from build123d import *

# Parameters (mm, degrees)
SKETCH3_RX          = 5.624926532
SKETCH3_RY          = 3.004692616
SKETCH3_RX_2        = 9.556829234
SKETCH3_RY_2        = 4.328681477
SKETCH3_RX_3        = 8.492460802
SKETCH3_RY_3        = 4.684720213
SKETCH3_RX_4        = 5.848490675
SKETCH3_RY_4        = 3.57108896
SKETCH3_RX_5        = 14.471517628
SKETCH3_RY_5        = 10.662983723
BOSS_EXTRUDE2_DEPTH = 2.5


with BuildPart() as part:
    # Sketch3 → Boss-Extrude2 (new body)
    with BuildSketch(Plane(origin=(0, 0, 0), x_dir=(1, 0, 0), z_dir=(0, 1, 0))):
        Polygon((10.338651831, 158.825979178), (13.264554689, 163.800014037), (45.578225854, 148.199099997), (73.311205528, 123.503793754), (73.311205528, 113.306124028), (70.253487054, 110.248405554), (70.253487054, 91.907219464), (73.927331416, 81.033815485), (86.933442966, 42.539886198), (86.933442966, 30.301657501), (81.461542635, 24.829757171), (81.461542635, -24.829757171), (86.933442966, -30.301657501), (86.933442966, -42.539886198), (73.927331416, -81.033815485), (70.253487054, -91.907219464), (70.253487054, -110.248405554), (73.311205528, -113.306124028), (73.311205528, -123.503793754), (45.578225854, -148.199099997), (13.264554689, -163.800014037), (10.338651831, -158.825979178), (-10.338651831, -158.825979178), (-13.264554689, -163.800014037), (-45.578225854, -148.199099997), (-73.311205528, -123.503793754), (-73.311205528, -113.306124028), (-70.253487054, -110.248405554), (-70.253487054, -91.907219464), (-73.927331416, -81.033815485), (-86.933442966, -42.539886198), (-86.933442966, -30.301657501), (-81.461542635, -24.829757171), (-81.461542635, 24.829757171), (-86.933442966, 30.301657501), (-86.933442966, 42.539886198), (-73.927331416, 81.033815485), (-70.253487054, 91.907219464), (-70.253487054, 110.248405554), (-73.311205528, 113.306124028), (-73.311205528, 123.503793754), (-45.578225854, 148.199099997), (-13.264554689, 163.800014037), (-10.338651831, 158.825979178), align=None)
        with Locations(Location((11.385123615, 149.68538673), (0, 0, 83.157226587))):
            Ellipse(SKETCH3_RX, SKETCH3_RY, mode=Mode.SUBTRACT)
        with Locations(Location((33.692455497, 82.363006755), (0, 0, 39.093858886))):
            Ellipse(SKETCH3_RX_2, SKETCH3_RY_2, mode=Mode.SUBTRACT)
        with Locations(Location((44.895501329, 74.018669169), (0, 0, 39.093858886))):
            Ellipse(SKETCH3_RX_3, SKETCH3_RY_3, mode=Mode.SUBTRACT)
        with Locations(Location((66.355525512, 66.446955434), (0, 0, 82.221640152))):
            Ellipse(SKETCH3_RX_4, SKETCH3_RY_4, mode=Mode.SUBTRACT)
        with Locations(Location((-66.355525512, 66.446955434), (0, 0, 97.778359848))):
            Ellipse(SKETCH3_RX_4, SKETCH3_RY_4, mode=Mode.SUBTRACT)
        with Locations(Location((-44.895501329, 74.018669169), (0, 0, 140.906141114))):
            Ellipse(SKETCH3_RX_3, SKETCH3_RY_3, mode=Mode.SUBTRACT)
        with Locations(Location((-33.692455497, 82.363006755), (0, 0, 140.906141114))):
            Ellipse(SKETCH3_RX_2, SKETCH3_RY_2, mode=Mode.SUBTRACT)
        with Locations(Location((-11.385123615, 149.68538673), (0, 0, 96.842773413))):
            Ellipse(SKETCH3_RX, SKETCH3_RY, mode=Mode.SUBTRACT)
        with Locations(Location((-11.385123615, -149.68538673), (0, 0, -96.842773413))):
            Ellipse(SKETCH3_RX, SKETCH3_RY, mode=Mode.SUBTRACT)
        with Locations(Location((-33.692455497, -82.363006755), (0, 0, -140.906141114))):
            Ellipse(SKETCH3_RX_2, SKETCH3_RY_2, mode=Mode.SUBTRACT)
        with Locations(Location((-44.895501329, -74.018669169), (0, 0, -140.906141114))):
            Ellipse(SKETCH3_RX_3, SKETCH3_RY_3, mode=Mode.SUBTRACT)
        with Locations(Location((-66.355525512, -66.446955434), (0, 0, -97.778359848))):
            Ellipse(SKETCH3_RX_4, SKETCH3_RY_4, mode=Mode.SUBTRACT)
        with Locations(Location((66.355525512, -66.446955434), (0, 0, -82.221640152))):
            Ellipse(SKETCH3_RX_4, SKETCH3_RY_4, mode=Mode.SUBTRACT)
        with Locations(Location((44.895501329, -74.018669169), (0, 0, -39.093858886))):
            Ellipse(SKETCH3_RX_3, SKETCH3_RY_3, mode=Mode.SUBTRACT)
        with Locations(Location((33.692455497, -82.363006755), (0, 0, -39.093858886))):
            Ellipse(SKETCH3_RX_2, SKETCH3_RY_2, mode=Mode.SUBTRACT)
        with Locations(Location((11.385123615, -149.68538673), (0, 0, -83.157226587))):
            Ellipse(SKETCH3_RX, SKETCH3_RY, mode=Mode.SUBTRACT)
        with Locations(Location((0, 0), (0, 0, 90))):
            Ellipse(SKETCH3_RX_5, SKETCH3_RY_5, mode=Mode.SUBTRACT)
        Polygon((5.834875923, 128.014628126), (5.834875923, 107.44522339), (9.270194242, 107.44522339), (10.662983723, 103.716266976), (20.757785776, 101.069910811), (32.198995676, 111.76010755), (32.198995676, 123.503793754), (24.907753398, 123.503793754), (13.841173073, 132.585606956), (9.270194242, 132.585606956), align=None, mode=Mode.SUBTRACT)
        Polygon((41.941351313, 39.789061162), (51.486619053, 54.160218526), (55.402714886, 54.160218526), (58.163676153, 51.399257259), (58.163676153, 43.187167337), (66.355525512, 28.46204058), (66.355525512, 24.072820104), (62.259600832, 17.90608076), (47.849651346, 18.166894335), (41.941351313, 27.187750764), align=None, mode=Mode.SUBTRACT)
        Polygon((-41.941351313, 27.187750764), (-41.941351313, 39.789061162), (-51.486619053, 54.160218526), (-55.402714886, 54.160218526), (-58.163676153, 51.399257259), (-58.163676153, 43.187167337), (-66.355525512, 28.46204058), (-66.355525512, 24.072820104), (-62.259600832, 17.90608076), (-47.849651346, 18.166894335), align=None, mode=Mode.SUBTRACT)
        Polygon((-9.270194242, 132.585606956), (-5.834875923, 128.014628126), (-5.834875923, 107.44522339), (-9.270194242, 107.44522339), (-10.662983723, 103.716266976), (-20.757785776, 101.069910811), (-32.198995676, 111.76010755), (-32.198995676, 123.503793754), (-24.907753398, 123.503793754), (-13.841173073, 132.585606956), align=None, mode=Mode.SUBTRACT)
        Polygon((-5.834875923, -128.014628126), (-5.834875923, -107.44522339), (-9.270194242, -107.44522339), (-10.662983723, -103.716266976), (-20.757785776, -101.069910811), (-32.198995676, -111.76010755), (-32.198995676, -123.503793754), (-24.907753398, -123.503793754), (-13.841173073, -132.585606956), (-9.270194242, -132.585606956), align=None, mode=Mode.SUBTRACT)
        Polygon((-41.941351313, -39.789061162), (-51.486619053, -54.160218526), (-55.402714886, -54.160218526), (-58.163676153, -51.399257259), (-58.163676153, -43.187167337), (-66.355525512, -28.46204058), (-66.355525512, -24.072820104), (-62.259600832, -17.90608076), (-47.849651346, -18.166894335), (-41.941351313, -27.187750764), align=None, mode=Mode.SUBTRACT)
        Polygon((41.941351313, -27.187750764), (41.941351313, -39.789061162), (51.486619053, -54.160218526), (55.402714886, -54.160218526), (58.163676153, -51.399257259), (58.163676153, -43.187167337), (66.355525512, -28.46204058), (66.355525512, -24.072820104), (62.259600832, -17.90608076), (47.849651346, -18.166894335), align=None, mode=Mode.SUBTRACT)
        Polygon((9.270194242, -132.585606956), (5.834875923, -128.014628126), (5.834875923, -107.44522339), (9.270194242, -107.44522339), (10.662983723, -103.716266976), (20.757785776, -101.069910811), (32.198995676, -111.76010755), (32.198995676, -123.503793754), (24.907753398, -123.503793754), (13.841173073, -132.585606956), align=None, mode=Mode.SUBTRACT)
    extrude(amount=BOSS_EXTRUDE2_DEPTH)


solid = part.part
Geometry check sheet. Reference: the model listing, model coordinates, mm. A direction names the side the tool comes from. Give positions to 0.01 mm unless a question says otherwise; leave off trailing zeros.
(1) Release check for a two-part mould opening along Z. For faces 3 (the flat face through (-29.65, 1.23, -155.89)), 4 (the flat face through (-18, 2.5, -2)), 5 (the flat face through (-59.251, 1.232, 136.024)), 6 (the flat face through (26.4, 1.23, -106.34)) record: released by +Z, released by -Z, zero draft, split by the parting line, or undercut.
From the geometry:
face 3: released by -Z
face 4: zero draft
face 5: released by +Z
face 6: undercut
(2) Thickness scan on L1, parallel to X at y = 0.2, z = 118.5; L2, parallel to X at y = 1.7, z = 41; L3, parallel to Z at x = -37, y = 0.9. Record the ranges inside material, lowest first.
From the geometry:
L1: x = -73.31 to -32.2, -5.83 to 5.83, 32.2 to 73.31
L2: x = -86.93 to -59.38, -42.75 to 42.75, 59.38 to 86.93
L3: z = -152.34 to -89, -79.49 to 79.49, 89 to 152.34
(3) Depth check by flat-ended pin: pin 1 Ø1.2 at (x, y) = (12, 1.5) entering from -Z; pin 2 Ø1.2 at (y, z) = (0.5, 120.5) entering from +X; pin 3 Ø0.8 at (y, z) = (0.5, -26.5) entering from -X. Enter the tip coordinate at first touch or a pass-through.
From the geometry:
pin 1: stops at z = -162.67
pin 2: stops at x = 73.31
pin 3: stops at x = -83.53
(4) Section check A-A on y = 0.7. Count the separate pieces of the cut face and the enclosed holes in it, then the cut area to 3 significant figures.
From the geometry:
separate pieces: 1
enclosed holes: 25
area: 39,300 mm2
(5) Set-up check for faces 1 (the flat face through (-59.64, 1.23, -135.68)), 2 (the flat face through (26.4, 1.23, 106.34)): record each of +Z, -Z, +X, -X, +Y, -Y from which the full face is reachable in a straight line by a thin tool's end or side.
From the geometry:
face 1: -Z, -X, +Y, -Y
face 2: +Y, -Y
